Could you check a few things on this model? Use its own coordinates, in mm. A direction names the side the tool comes from. Coordinates: 2 decimals unless noted, no trailing zeros. Write each loop counter-clockwise with the first axis right and the second up, starting at its lowest first coordinate (ties: lowest second). Pieces come first, ordered by that corner, then holes. Notation, with made-up numbers: (-15.75, -8.75) - (30.25, -8.75) arc R19 ccw to (30.25, 6.25) - close; hole circle Ø5 at (26, -12). An arc over 180 degrees is marked (long way). Write item = value, one per line. Start each with the question number.
```python
from build123d import *

# Parameters (mm, degrees)
SKETCH1_W                       = 44.45
SKETCH1_H                       = 52.7704812
EXTRUDE1_DEPTH                  = 12.5
M4X0_7_TAPPED_HOLE2_D           = 3.3
CBORE_FOR_M6_SBHCS1_D           = 6.6
CBORE_FOR_M6_SBHCS1_CBORE_D     = 11.5
CBORE_FOR_M6_SBHCS1_CBORE_DEPTH = 8.3
SKETCH6_W                       = 44.45
SKETCH6_H                       = 22.583276864
EXTRUDE2_DEPTH                  = 8.255
SKETCH7_W                       = 44.45
SKETCH7_H                       = 19.975275
EXTRUDE3_DEPTH                  = 4
SKETCH8_W                       = 9.398
SKETCH8_H                       = 22.583276864
CUT_EXTRUDE1_DEPTH              = 2.54
FILLET1_R                       = 1.5875
M4X0_7_TAPPED_HOLE3_D           = 3.3


with BuildPart() as part:
    # Sketch1 → Extrude1 (new body)
    with BuildSketch(Plane(origin=(0, 0, 0), x_dir=(1, 0, 0), z_dir=(0, 1, 0))):
        Rectangle(SKETCH1_W, SKETCH1_H)
    extrude1 = extrude(amount=EXTRUDE1_DEPTH)

    # M4x0.7 Tapped Hole2 (through all)
    with Locations(Plane(origin=(0, 12.5, 0), x_dir=(-1, 0, 0), z_dir=(0, 1, 0))):
        with Locations((9.525000018, -19.236265325), (-9.525000018, -19.236265325)):
            Hole(M4X0_7_TAPPED_HOLE2_D / 2)

    # CBORE for M6 SBHCS1 (through all)
    with Locations(Plane(origin=(0, 12.5, 0), x_dir=(-1, 0, 0), z_dir=(0, 1, 0))):
        with Locations((15.24, 13.8852406), (-9.76, 13.8852406)):
            cbore_for_m6_sbhcs1 = CounterBoreHole(CBORE_FOR_M6_SBHCS1_D / 2, CBORE_FOR_M6_SBHCS1_CBORE_D / 2, CBORE_FOR_M6_SBHCS1_CBORE_DEPTH)

    # Mirror1: Extrude1, CBORE for M6 SBHCS1 across plane
    add(extrude1.mirror(Plane(origin=(-22.225, 12.5, 26.3852406), x_dir=(1, 0, 0), z_dir=(0, 0, -1))))
    add(cbore_for_m6_sbhcs1.mirror(Plane(origin=(-22.225, 12.5, 26.3852406), x_dir=(1, 0, 0), z_dir=(0, 0, -1))), mode=Mode.SUBTRACT)

    # Sketch6 → Extrude2 (cut)
    with BuildSketch(Plane.XZ):
        with Locations((0, 67.864083368)):
            Rectangle(SKETCH6_W, SKETCH6_H)
    extrude(amount=-EXTRUDE2_DEPTH, mode=Mode.SUBTRACT)

    # Sketch7 → Extrude3 (cut)
    with BuildSketch(Plane.XZ):
        with Locations((0, -16.3976031)):
            Rectangle(SKETCH7_W, SKETCH7_H)
    extrude(amount=-EXTRUDE3_DEPTH, mode=Mode.SUBTRACT)

    # Sketch8 → Cut-Extrude1 (cut)
    with BuildSketch(Plane.XZ.offset(-8.255)):
        with Locations((-15.2432004, 67.864083368)):
            Rectangle(SKETCH8_W, SKETCH8_H)
    extrude(amount=-CUT_EXTRUDE1_DEPTH, mode=Mode.SUBTRACT)

    # Fillet1
    fillet1_edges = [part.edges().sort_by_distance(p)[0] for p in [
        (-10.5442004, 9.525, 56.572444936),
        (-19.9422004, 10.795, 67.864083368),
        (-19.9422004, 9.525, 56.572444936),
        (-10.5442004, 10.795, 67.864083368),
        (-15.2432004, 10.795, 56.572444936),
    ]]
    fillet(fillet1_edges, radius=FILLET1_R)

    # M4x0.7 Tapped Hole3 (through all)
    with Locations(Plane(origin=(0, 12.5, 0), x_dir=(-1, 0, 0), z_dir=(0, 1, 0))):
        with Locations((-9.524999982, 71.7115406), (8.596896608, 71.7115406)):
            Hole(M4X0_7_TAPPED_HOLE3_D / 2)


solid = part.part
```
1) Suppose I cut it at A-A on x = -15.24. Please give me the cut outline in (y, z) (1 decimal), plus the area to 3 significant figures.
2) If I drill on probe 1 along X at (y, z) = (10.25, 19) (3 decimals); probe 2 along X at (y, z) = (7.5, 41) (3 decimals); probe 3 along Y at (x, z) = (-13, 19), over which ranges is the centre line in solid material (lowest first)? Write a range as [from, to].
3) Which directions (+Z, -Z, +X, -X, +Y, -Y) give clear straight access to the entire face, cutting with the end or side of a thin tool? Please do faces 3 (the flat face through (-15, 10.795, 69)), 4 (the flat face through (0, 2, -6.41)), 5 (the cylindrical face through (7.33, 2.07, 16.12)), 6 (the flat face through (5, 8.255, 68)), 7 (the cylindrical face through (-14.491, 8.408, 33.184)).
4) Suppose I cut it at C-C on y = 5.75. Please give me the cut outline in (x, z) (3 decimals), plus the area to 3 significant figures.
5) Suppose I cut it at B-B on x = 9.76. State how many separate pieces and enclosed holes the cut face has, plus the area to 3 significant figures.
6) Thinking about a two-plate mould opening in X: for faces 1 (the cylindrical face through (10.509, 8.408, 19.586)), 2 (the flat face through (0, 4, -16)), which applies, +X half, -X half, draft (parallel to the pull), parting line (faces both ways), or undercut?
7) For P1, Ø10.5, axis at x = -15.24, z = 13.89, coming from the +Y side; P2, Ø2, axis at x = -9.53, z = -19.24, coming from the -Y side; P3, Ø6, axis at x = 5, z = -19.5, coming from the -Y side, each with a flat end and sliding along its axis, tell me the tip position at first contact or that it passes through.
8) Suppose I cut it at D-D on x = -0.5. Please give me the cut outline in (y, z) (3 decimals), plus the area to 3 significant figures.
Reply:
q1.outline = (0, -6.4) - (4, -6.4) - (4, -26.4) - (12.5, -26.4) - (12.5, 8.1) - (4.2, 8.1) - (4.2, 10.6) - (0, 10.6) - close; (0, 17.2) - (4.2, 17.2) - (4.2, 19.6) - (12.5, 19.6) - (12.5, 33.1) - (4.2, 33.1) - (4.2, 35.6) - (0, 35.6) - close; (0, 42.2) - (4.2, 42.2) - (4.2, 44.6) - (12.5, 44.6) - (12.5, 79.2) - (10.8, 79.2) - (10.8, 58.2) arc R1.6 cw to (9.2, 56.6) - (0, 56.6) - close
q1.area = 750 mm^2
q2.probe_1 = [-22.225, -17.867], [-12.613, 7.133], [12.387, 22.225]
q2.probe_2 = [-22.225, -20.587], [-9.893, 4.413], [15.107, 22.225]
q2.probe_3 = [0, 4.2]
q3.face_3 = +Z, -Y
q3.face_4 = -Z, +X, -X, -Y
q3.face_5 = +Y, -Y
q3.face_6 = +Z, +X, -X, -Y
q3.face_7 = +Y
q4.outline = (-22.225, -26.385) - (22.225, -26.385) - (22.225, 56.572) - (-22.225, 56.572) - close; hole circle Ø11.5 at (-15.24, 13.885); hole circle Ø11.5 at (-15.24, 38.885); hole circle Ø3.3 at (-9.525, -19.236); hole circle Ø11.5 at (9.76, 13.885); hole circle Ø11.5 at (9.76, 38.885); hole circle Ø3.3 at (9.525, -19.236)
q4.area = 3,250 mm^2
q5.separate_pieces = 5
q5.enclosed_holes = 0
q5.area = 765 mm^2
q6.face_1 = undercut
q6.face_2 = draft
q7.P1 = 4.2
q7.P2 = through
q7.P3 = 4
q8.outline = (0, -6.41) - (4, -6.41) - (4, -26.385) - (12.5, -26.385) - (12.5, 79.156) - (8.255, 79.156) - (8.255, 56.572) - (0, 56.572) - close
q8.area = 1,050 mm^2
